```python
from build123d import *

# Parameters (mm, degrees)
SKETCH1_W            = 151.5
SKETCH1_H            = 151.5
BOSS_EXTRUDE1_DEPTH  = 2
SKETCH2_R            = 14.75
CUT_EXTRUDE2_DEPTH   = 2
LPATTERN1_COUNT      = 4
LPATTERN1_PITCH      = 33.5
LPATTERN1_COUNT_DIR2 = 4
LPATTERN1_PITCH_DIR2 = 33.5
SKETCH3_W            = 151.5
SKETCH3_H            = 151.5
BOSS_EXTRUDE2_DEPTH  = 10
SKETCH5_W            = 148.5
SKETCH5_H            = 148.5
CUT_EXTRUDE4_DEPTH   = 10
SKETCH8_R            = 3.5
BOSS_EXTRUDE4_DEPTH  = 10
LPATTERN2_COUNT      = 2
LPATTERN2_PITCH      = 105
LPATTERN2_COUNT_DIR2 = 2
LPATTERN2_PITCH_DIR2 = 105


with BuildPart() as part:
    # Sketch1 → Boss-Extrude1 (new body)
    with BuildSketch(Plane(origin=(0, 0, 0), x_dir=(1, 0, 0), z_dir=(0, 1, 0))):
        with Locations((75.75, 75.75)):
            Rectangle(SKETCH1_W, SKETCH1_H)
    extrude(amount=BOSS_EXTRUDE1_DEPTH)

    # Sketch2 → Cut-Extrude2 (cut)
    with BuildSketch(Plane(origin=(0, 0, 0), x_dir=(1, 0, 0), z_dir=(0, 1, 0))):
        with Locations((34.25, 34.25)):
            Circle(SKETCH2_R)
    cut_extrude2 = extrude(amount=CUT_EXTRUDE2_DEPTH, mode=Mode.SUBTRACT)

    # LPattern1: Cut-Extrude2 4 × 4
    with Locations(*[(i * LPATTERN1_PITCH, 0, -j * LPATTERN1_PITCH_DIR2) for i in range(LPATTERN1_COUNT) for j in range(LPATTERN1_COUNT_DIR2) if (i, j) != (0, 0)]):
        add(cut_extrude2, mode=Mode.SUBTRACT)

    # Sketch3 → Boss-Extrude2 (add)
    with BuildSketch(Plane(origin=(0, 0, 0), x_dir=(1, 0, 0), z_dir=(0, 1, 0))):
        with Locations((75.75, 75.75)):
            Rectangle(SKETCH3_W, SKETCH3_H)
    extrude(amount=-BOSS_EXTRUDE2_DEPTH)

    # Sketch5 → Cut-Extrude4 (cut)
    with BuildSketch(Plane(origin=(0, 0, 0), x_dir=(1, 0, 0), z_dir=(0, 1, 0))):
        with Locations((77.25, 77.25)):
            Rectangle(SKETCH5_W, SKETCH5_H)
    extrude(amount=-CUT_EXTRUDE4_DEPTH, mode=Mode.SUBTRACT)

    # Sketch8 → Boss-Extrude4 (add)
    with BuildSketch(Plane(origin=(0, 0, 0), x_dir=(1, 0, 0), z_dir=(0, 1, 0))):
        with Locations((13, 13)):
            Circle(SKETCH8_R)
    boss_extrude4 = extrude(amount=-BOSS_EXTRUDE4_DEPTH)

    # LPattern2: Boss-Extrude4 2 × 2
    with Locations(*[(j * LPATTERN2_PITCH_DIR2, 0, -i * LPATTERN2_PITCH) for i in range(LPATTERN2_COUNT) for j in range(LPATTERN2_COUNT_DIR2) if (i, j) != (0, 0)]):
        add(boss_extrude4)


solid = part.part
```
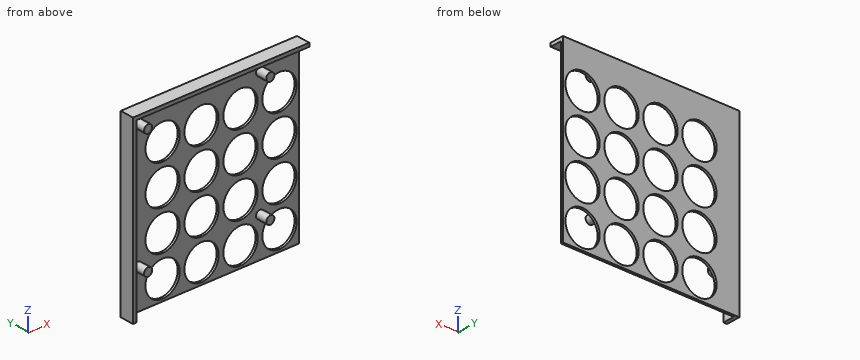
Source: CAD feature listing. Evaluate the final solid. Frame: model axes, mm. Coordinates: 2 decimals unless noted, no trailing zeros. Loops run counter-clockwise (first coordinate to the right, second up) from the corner with the lowest first, then second, coordinate; pieces in that order, holes last. Notation, with made-up numbers: M 55,-21 L 104,-21 A23 cw 104,9 Z; hole C -4,-39.75 d2. An arc over 180 degrees is marked long. Use a Markdown table: item, result. Add a question column.
Q1. Section query D-D, the plane x = 118. Return loops of the section in (y, z), and give its area (3 significant figures).
Q2. Section query B-B, the plane y = -4. Return loops of the section in (x, z), and give its area (3 significant figures).
Q3. Section query C-C, the plane z = -67.75. Return loops of the section in (x, y).
Q4. Section query A-A, the plane x = 67.75. Return loops of the section in (y, z), and give its area (3 significant figures).
Q5. First-contact query: pin 1 (8 mm diameter, centred on x = 88.5, z = -112.5, fed in from -Y). Flat tip, straight axial feed; report the tip coordinate or a pass-through.
Q6. Material intervals for L1, parallel to X at y = 1.5, z = -101.25; L2, parallel to Z at x = 67.75, y = 1.05; L3, parallel to Z at x = 14.5, y = -4, sorted ascending.
Result:
| question | item | result |
|---|---|---|
| 1 | outline | M -10,-121.5 L 0,-121.5 L 0,-151.5 L 2,-151.5 L 2,0 L -10,0 L -10,-3 L 0,-3 L 0,-9.5 L -10,-9.5 L -10,-16.5 L 0,-16.5 L 0,-114.5 L -10,-114.5 Z |
| 1 | area | 473 mm2 |
| 2 | outline | M 0,-151.5 L 3,-151.5 L 3,-3 L 151.5,-3 L 151.5,0 L 0,0 Z; C 13,-118 d7; C 13,-13 d7; C 118,-118 d7; C 118,-13 d7 |
| 2 | area | 1,050 mm2 |
| 3 | outline | M 0,-10 L 3,-10 L 3,0 L 19.5,0 L 19.5,2 L 0,2 Z; M 49,0 L 53,0 L 53,2 L 49,2 Z; M 82.5,0 L 86.5,0 L 86.5,2 L 82.5,2 Z; M 116,0 L 120,0 L 120,2 L 116,2 Z; M 149.5,0 L 151.5,0 L 151.5,2 L 149.5,2 Z |
| 4 | outline | M -10,-3 L 0,-3 L 0,-19.5 L 2,-19.5 L 2,0 L -10,0 Z; M 0,-151.5 L 2,-151.5 L 2,-149.5 L 0,-149.5 Z; M 0,-120 L 2,-120 L 2,-116 L 0,-116 Z; M 0,-86.5 L 2,-86.5 L 2,-82.5 L 0,-82.5 Z; M 0,-53 L 2,-53 L 2,-49 L 0,-49 Z |
| 4 | area | 97.0 mm2 |
| 5 | pin 1 | stops at y = 0 |
| 6 | L1 | x = 0 to 19.5, 49 to 53, 82.5 to 86.5, 116 to 120, 149.5 to 151.5 |
| 6 | L2 | z = -151.5 to -149.5, -120 to -116, -86.5 to -82.5, -53 to -49, -19.5 to 0 |
| 6 | L3 | z = -121.16 to -114.84, -16.16 to -9.84, -3 to 0 |
